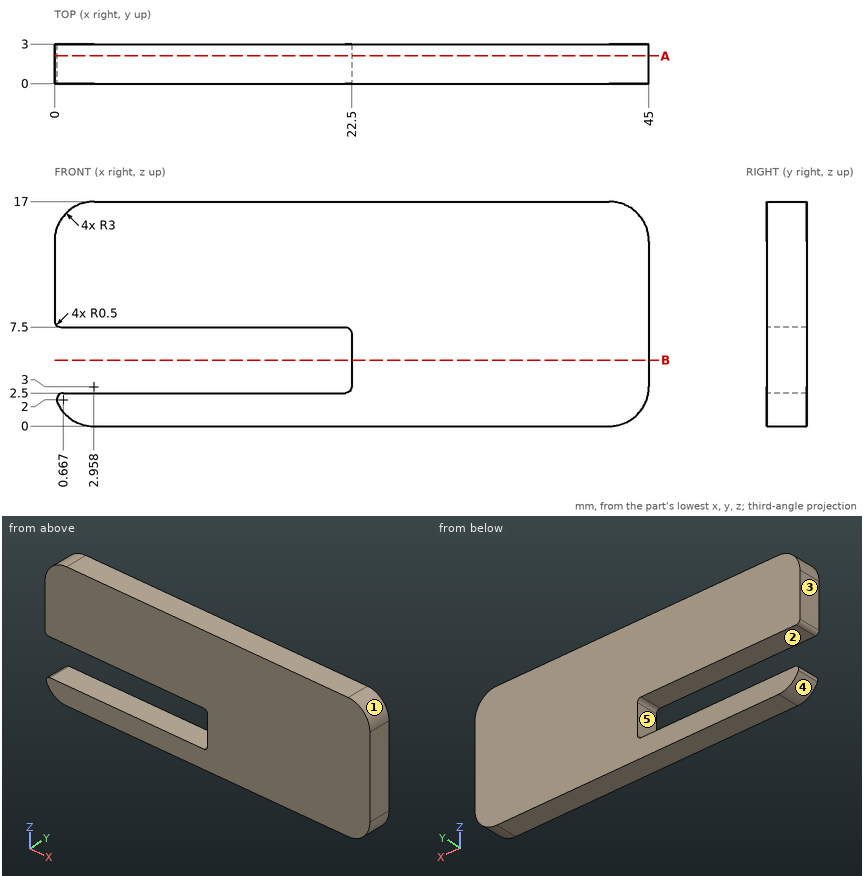
Part print with two shaded views. Sizes in mm from the minimum x, y, z corner. A direction names the side the tool comes from. Round coordinates to 2 decimals unless told otherwise and drop trailing zeros. Order: outer loops, then holes, each group sorted by start corner. A loop starts at its lowest first (then second) coordinate and runs counter-clockwise, first axis right, second up. Notation, with made-up numbers: (0, 39.5) -> (18, 39.5) arc R20 ccw to (18, 67.5) -> close; hole circle Ø8 at (49, -8). An arc over 180 degrees is marked (long way). Write each question's results on one line, items separated by ' | '.
1. Cut at B-B (z = 5). Give the cut face in (x, y), plus the area to 3 significant figures.
Findings below:
outline: (22.5, 0) -> (45, 0) -> (45, 3) -> (22.5, 3) -> close | area: 67.5 mm²
2. Wall check: line 1 along Z through (x, y) = (11, 1.8); line 2 along X through (y, z) = (0.9, 5.25); line 3 along X through (y, z) = (0.2, 16) (1 decimal). Give the ranges that are in metal, low to high. Write a range as [from, to].
Findings below:
line 1: z = [0, 2.5], [7.5, 17] | line 2: x = [22.5, 45] | line 3: x = [0.8, 44.2]
3. 3-axis set-ups, long thin cutter, end or side, ignore diameter. For the marked faces 4 and 5: which of +Z, -Z, +X, -X, +Y, -Y reach the whole face in a straight line?
Findings below:
face 4: -Z, -X, +Y, -Y | face 5: -X, +Y, -Y
4. Pull direction Z, two halves, no side cores. Call the marked faces 1, 2 and 3: pulls with the +Z half, pulls with the -Z half, needs draft (parallel to the pull), parting line crosses it, or undercut.
Findings below:
face 1: pulls with the +Z half | face 2: undercut | face 3: needs draft
5. Cut at A-A (y = 2.1). Give the cut face in (x, z).
Findings below:
outline: (0, 8) arc R0.5 ccw to (0.5, 7.5) -> (22, 7.5) arc R0.5 cw to (22.5, 7) -> (22.5, 3) arc R0.5 cw to (22, 2.5) -> (0.67, 2.5) arc R0.5 ccw to (0.21, 1.8) arc R3 ccw to (2.96, 0) -> (42, 0) arc R3 ccw to (45, 3) -> (45, 14) arc R3 ccw to (42, 17) -> (3, 17) arc R3 ccw to (0, 14) -> close
6. Flat gauge pins, fed straight in: P1, Ø4, axis at x = 39.5, z = 8, coming from the -Y side; P2, Ø1.5, axis at y = 1, z = 4.5, coming from the -X side. Where does each tip first touch, or does it go through?
Findings below:
P1: stops at y = 0 | P2: stops at x = 22.5
